```python
from build123d import *

# Parameters (mm, degrees)
SKETCH1_R           = 19.05
BOSS_EXTRUDE1_DEPTH = 5.08
SKETCH2_R           = 12.7
BOSS_EXTRUDE2_DEPTH = 19.05
CUT_EXTRUDE1_REACH  = 38.167
SKETCH3_R           = 8.89


with BuildPart() as part:
    # Sketch1 → Boss-Extrude1 (new body)
    with BuildSketch(Plane.XY):
        Circle(SKETCH1_R)
    extrude(amount=-BOSS_EXTRUDE1_DEPTH)

    # Sketch2 → Boss-Extrude2 (add)
    with BuildSketch(Plane.XY):
        with Locations(Location((0, 0, 0), (0, 0, 180))):
            Circle(SKETCH2_R)
    extrude(amount=BOSS_EXTRUDE2_DEPTH)

    # Sketch3 → Cut-Extrude1 (cut, up to next)
    with BuildSketch(Plane.XY.offset(19.05), mode=Mode.PRIVATE) as cut_extrude1_sk1:
        Circle(SKETCH3_R)
    cut_extrude1_tool1 = extrude(cut_extrude1_sk1.sketch, amount=-CUT_EXTRUDE1_REACH, mode=Mode.PRIVATE) & part.part
    add(cut_extrude1_tool1.solids().sort_by_distance((0, 0, 19.05))[0], mode=Mode.SUBTRACT)


solid = part.part
```
Here's how the part is built. I have some questions about the finished solid (model axes, mm). A direction names the side the tool comes from. Round coordinates to 2 decimals unless told otherwise and drop trailing zeros. Order: outer loops, then holes, each group sorted by start corner. A loop starts at its lowest first (then second) coordinate and runs counter-clockwise, first axis right, second up. Notation, with made-up numbers: M 38,39.5 L 76,39.5 A14 ccw 76,52.5 Z; hole C -2,49 d2. An arc over 180 degrees is marked long. Answer in a Markdown table with one row per item.
Item 1: Thinking about a two-plate mould opening in Y: for faces 1 (the face through (8.2, -4, -5.08)), 2 (the face through (-15.12, -11.59, -2.5)), 3 (the face through (-1.93, -8.68, 7.15)), which applies, +Y half, -Y half, draft (parallel to the pull), parting line (faces both ways), or undercut?
A:
| item | result |
|---|---|
| face 1 | draft |
| face 2 | parting line |
| face 3 | undercut |
Item 2: Imagine slicing it at D-D, the plane y = -11. Write out the boundary of the cut face in (x, z), and give its area (3 significant figures).
A:
| item | result |
|---|---|
| outline | M -15.55,-5.08 L 15.55,-5.08 L 15.55,0 L 6.35,0 L 6.35,19.05 L -6.35,19.05 L -6.35,0 L -15.55,0 Z |
| area | 400 mm2 |
Item 3: I'm going to push flat-ended pins straight in: pin 1 (12 mm diameter, centred on y = -3, z = -1.5, fed in from +X); pin 2 (5 mm diameter, centred on y = -6.5, z = 3, fed in from +X); pin 3 (8 mm diameter, centred on x = 0, z = 7, fed in from +Y); pin 4 (2 mm diameter, centred on y = -11, z = 11, fed in from -X). Where does each tip first touch, or does it pass through?
A:
| item | result |
|---|---|
| pin 1 | stops at x = 19.05 |
| pin 2 | stops at x = 12.05 |
| pin 3 | stops at y = 12.7 |
| pin 4 | stops at x = -7.83 |
Item 4: Imagine slicing it at C-C, the plane z = -1.25. Write out the boundary of the cut face in (x, y).
A:
| item | result |
|---|---|
| outline | C 0,0 d38.1; hole C 0,0 d17.78 |
Item 5: Imagine slicing it at A-A, the plane y = 0. Write out the boundary of the cut face in (x, z).
A:
| item | result |
|---|---|
| outline | M -19.05,-5.08 L -8.89,-5.08 L -8.89,19.05 L -12.7,19.05 L -12.7,0 L -19.05,0 Z; M 8.89,-5.08 L 19.05,-5.08 L 19.05,0 L 12.7,0 L 12.7,19.05 L 8.89,19.05 Z |
Item 6: If I drill on L1, parallel to Y at x = 0, z = 12.75; L2, parallel to Z at x = 9, y = 13; L3, parallel to Y at x = -3, z = 13.25, over which ranges is the centre line in solid material (lowest first)? Write a range as from..to.
A:
| item | result |
|---|---|
| L1 | y = -12.7..-8.89, 8.89..12.7 |
| L2 | z = -5.08..0 |
| L3 | y = -12.34..-8.37, 8.37..12.34 |
Item 7: For faces 4 (the face through (-5.86, 11.267, 9.392)), 5 (the face through (9, 3, 19.05)), which set-ups out of +Z, -Z, +X, -X, +Y, -Y let a thin tool reach every point of the face, with its end or its side?
A:
| item | result |
|---|---|
| face 4 | +Z |
| face 5 | +Z, +X, -X, +Y, -Y |
